Autodesk Inventor part; units mm, degrees
ref_plane "YZ Plane" through (0, 0, 0) normal (1, 0, 0) x (0, 1, 0)
ref_plane "XZ Plane" through (0, 0, 0) normal (0, 1, 0) x (-1, 0, 0)
ref_plane "XY Plane" through (0, 0, 0) normal (0, 0, 1) x (1, 0, 0)
sketch "Sketch1" plane through (0, 0, 0) normal (0, 0, 1) x (1, 0, 0)
  line L0 (0, 0) -> (8, 0)
  line L1 (8, 0) -> (8, 4)
  line L2 (8, 4) -> (0, 4)
  line L3 (0, 4) -> (0, 0)
  dimension "d0" = 8
  dimension "d1" = 4
extrude "Extrusion1" add sketch "Sketch1" along normal blind 26
sketch "Sketch3" plane through (8, 0, 0) normal (1, 0, 0) x (0, 0, -1)
  line L0 (0, 0) -> (0, 4)
  line L1 (-26, 0) -> (-26, 4)
  line L2 (0, 0) -> (-26, 0)
  arc A0 (-22.8, 0) -> (-26, 3) centre (-26.6879, -0.9404) ccw
  arc A1 (0, 3) -> (-3.2, 0) centre (0.6879, -0.9404) ccw
  dimension "d14" = 4
  dimension "d15" = 3.2
  dimension "d16" = 1
extrude "Extrusion2" cut sketch "Sketch3" against normal up to next
ref_plane "Work Plane1" through (0, 0, 3.2) normal (0, 0, -1) x (-1, 0, 0)
sketch "Sketch4" plane through (0, 0, 3.2) normal (0, 0, -1) x (-1, 0, 0)
  line L0 (0, 0) -> (-8, 0)
  line L1 (-8, 0) -> (0, 0)
  arc A0 (-5.6, 0) -> (-2.4, 0) centre (-4, 1.2) ccw
  line L2 (-8, 0) -> (-8, 3)
  line L3 (-5.6, 0) -> (-2.4, 0)
  dimension "d20" = 2
  dimension "d21" = 4
  dimension "d22" = 1.2
extrude "Extrusion3" add sketch "Sketch4" against normal blind 19.6
sketch "Sketch2" plane through (0, 4, 0) normal (0, 1, 0) x (1, 0, 0)
  line L0 (8, -26) -> (0, -26)
  line L1 (8, 0) -> (8, -26)
  point P0 (4, -7.5)
  point P1 (4, -18.5)
  dimension "d4" = 11
  dimension "d5" = 7.5
  dimension "d6" = 4
hole "Hole1" at (4, 4, 7.5) at (4, 4, 18.5) direction (0, -1, 0) diameter 4.5 end through all
properties part number "OfflineBowdenExtruderSpringHandle" material "ABS Plastic"
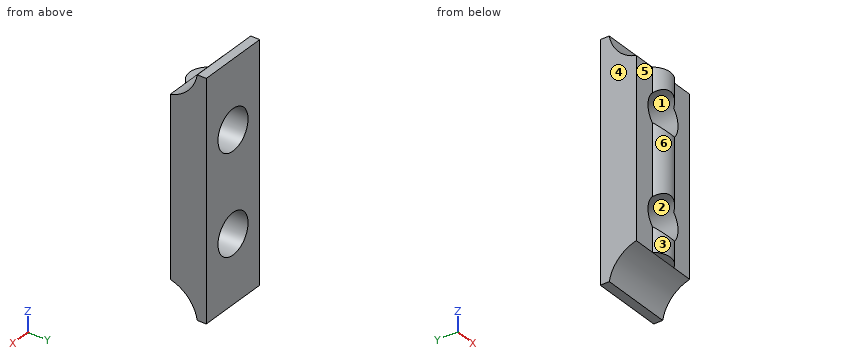
Could you check a few things on this model? Use its own coordinates, in mm. Face numbers are marked on the shaded views. A direction names the side the tool comes from. Coordinates: 2 decimals unless noted, no trailing zeros. Loops run counter-clockwise (first coordinate to the right, second up) from the corner with the lowest first, then second, coordinate; pieces in that order, holes last. Notation, with made-up numbers: M 74,-2 L 80,-2 A24 ccw 80,25 Z; hole C 19,74 d7. An arc over 180 degrees is marked long. Put each result on its own line as item: value. Start each with the question number.
(1) Thinking about a two-plate mould opening in X: for the marked faces 1, 2, 3 and 4, which applies, pulls with the +X half, pulls with the -X half, needs draft (parallel to the pull), parting line crosses it, or undercut?
(2) Suppose I cut it at A-A on x = 4. Please give me the cut outline in (y, z), then the cut area to 3 significant figures.
(3) For the marked faces 5 and 6, which set-ups out of +Z, -Z, +X, -X, +Y, -Y let a thin tool reach every point of the face, with its end or its side?
(4) Suppose I cut it at B-B on z = 7.5. Please give me the cut outline in (x, y), then the cut area to 3 significant figures.
(5) Will these pins go through, and if not, where does the flat tip stop? P1, Ø2.5, axis at x = 1, z = 14.5, coming from the -Y side; P2, Ø2, axis at x = 4, y = 0, coming from the -Z side; P3, Ø4, axis at x = 4, z = 18.5, coming from the +Y side.
(6) Suppose I cut it at C-C on y = -0.4. Please give me the cut outline in (x, z), then the cut area to 3 significant figures.
(7) I need wall thicknesses on line 1 (X direction, y = 1.9, z = 7.5); line 2 (Z direction, x = 4, y = 1); line 3 (Z direction, x = 4, y = 0.7). Which ranges of each line are inside material? Lowest first, please. Write a range as from..to.
(8) Suppose I cut it at D-D on y = 3.6. Please give me the cut outline in (x, z).
Solutions:
1. face 1: undercut
1. face 2: undercut
1. face 3: parting line crosses it
1. face 4: pulls with the -X half
2. outline: M -0.8,3.2 L 0,3.2 A4 cw 3,0 L 4,0 L 4,5.25 L -0.8,5.25 Z; M -0.8,9.75 L 4,9.75 L 4,16.25 L -0.8,16.25 Z; M -0.8,20.75 L 4,20.75 L 4,26 L 3,26 A4 cw 0,22.8 L -0.8,22.8 Z
2. area: 63.0 mm2
3. face 5: +Z, -Z, -X, -Y
3. face 6: +Z, -Z, -Y
4. outline: M 0,0 L 1.75,0 L 1.75,4 L 0,4 Z; M 6.25,0 L 8,0 L 8,4 L 6.25,4 Z
4. area: 14.0 mm2
5. P1: stops at y = 0
5. P2: stops at z = 2.81
5. P3: passes through
6. outline: M 2.8,3.2 L 5.2,3.2 L 5.2,5.6 A2.25 cw 2.8,5.6 Z; M 2.8,9.4 A2.25 cw 5.2,9.4 L 5.2,16.6 A2.25 cw 2.8,16.6 Z; M 2.8,20.4 A2.25 cw 5.2,20.4 L 5.2,22.8 L 2.8,22.8 Z
6. area: 26.5 mm2
7. line 1: x = 0..1.75, 6.25..8
7. line 2: z = 2.81..5.25, 9.75..16.25, 20.75..23.19
7. line 3: z = 2.96..5.25, 9.75..16.25, 20.75..23.04
8. outline: M 0,0 L 8,0 L 8,26 L 0,26 Z; hole C 4,7.5 d4.5; hole C 4,18.5 d4.5
